Part model, mm, in its own coordinate system. Face numbers are marked on the shaded views. A direction names the side the tool comes from. Give positions to 0.01 mm unless a question says otherwise; leave off trailing zeros. Order: outer loops, then holes, each group sorted by start corner. A loop starts at its lowest first (then second) coordinate and runs counter-clockwise, first axis right, second up. Notation, with made-up numbers: (3, -11.5) - (28, -11.5) arc R21 cw to (28, 4.5) - close; hole circle Ø7 at (-21, -15). An arc over 180 degrees is marked (long way). One line per item, written item: value.
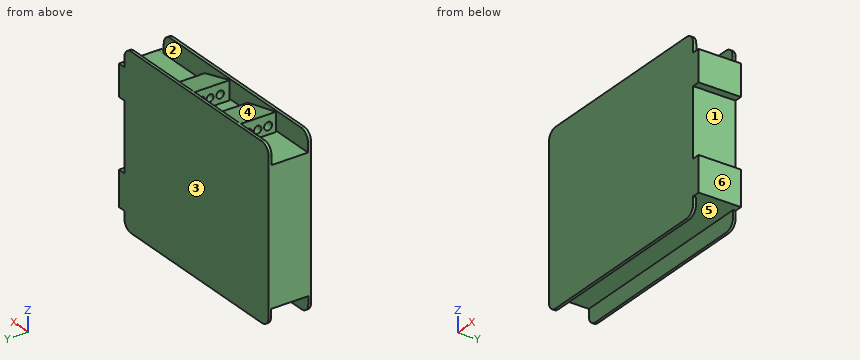
```python
from build123d import *

# Parameters (mm, degrees)
F1_DEPTH  = 22.5
F2_W      = 19.3578329636
F2_H      = 6.3240909576
F2_H_2    = 5.0115762651
F2_W_2    = 19.7066257242
F2_H_3    = 3.8353008032
F2_H_4    = 6.6283914447
F3_DEPTH  = 155.21203
F5_DEPTH  = 18.63889
F6_R      = 2.0341510362
F6_R_2    = 1.9663944792
F6_R_3    = 2.1232474026
F7_DEPTH  = 10
F8_R      = 2.0166596657
F8_R_2    = 1.8228540719
F8_R_3    = 1.9926186892
F9_DEPTH  = 10
F11_DEPTH = 5.64108
F13_DEPTH = 40.33136
F12_W     = 4
F12_H     = 18.4578578919
F12_H_2   = 17.5
F14_DEPTH = 25
F16_W     = 1.5692119678
F16_H     = 22.5
F17_DEPTH = 78.97005
F18_DEPTH = 25
F19_DEPTH = 25


with BuildPart() as f1:
    # F0 (on Front) → F1 (new body)
    with BuildSketch(Plane.XZ):
        with BuildLine():
            ThreePointArc((-43.9944155514, -30.0488834083), (-42.5299494574, -33.5844173142), (-38.9944155514, -35.0488834083))
            Line((-38.9944155514, -35.0488834083), (59.0055844486, -35.0488834083))
            ThreePointArc((59.0055844486, -35.0488834083), (62.5411183545, -33.5844173142), (64.0055844486, -30.0488834083))
            Line((64.0055844486, -30.0488834083), (64.0055844486, 49.9511165917))
            ThreePointArc((64.0055844486, 49.9511165917), (62.5411183545, 53.4866504976), (59.0055844486, 54.9511165917))
            Line((59.0055844486, 54.9511165917), (-38.9944155514, 54.9511165917))
            ThreePointArc((-38.9944155514, 54.9511165917), (-42.5299494574, 53.4866504976), (-43.9944155514, 49.9511165917))
            Line((-43.9944155514, 49.9511165917), (-43.9944155514, -30.0488834083))
        make_face()
    extrude(amount=F1_DEPTH)

    # F2 (on face) → F3 (cut)
    with BuildSketch(Plane(origin=(-43.9944155514, 0, 0), x_dir=(0, -1, 0), z_dir=(-1, 0, 0))):
        with Locations((11.1899548792, 53.1131620705)):
            Rectangle(F2_W, F2_H)
        with Locations((11.1899548792, 47.4453284591)):
            Rectangle(F2_W, F2_H_2)
        with Locations((11.1899542389, -28.1312330067)):
            Rectangle(F2_W_2, F2_H_3)
        with Locations((11.1899542389, -33.3630791306)):
            Rectangle(F2_W_2, F2_H_4)
    extrude(amount=-F3_DEPTH, mode=Mode.SUBTRACT)

    # F4 (on face) → F5 (join)
    with BuildSketch(Plane.XZ.offset(1.5110383974)):
        Polygon((0, 49.9453284591), (-21.0268571973, 54.9511165917), (-21.0268571973, 44.9395403266), (0, 44.9395403266), align=None)
        Polygon((32.1980565786, 49.9453284591), (13.5992644355, 54.9511165917), (13.5992644355, 44.9395403266), (32.1980565786, 44.9395403266), align=None)
    extrude(amount=F5_DEPTH)

    # F6 (on face) → F7 (cut)
    with BuildSketch(Plane(origin=(-21.0268571973, 0, 0), x_dir=(0, -1, 0), z_dir=(-1, 0, 0))):
        with Locations((5.4616648704, 49.1789467633)):
            Circle(F6_R)
        with Locations((10.4407919571, 49.1789467633)):
            Circle(F6_R_2)
        with Locations((15.9926619381, 49.1789467633)):
            Circle(F6_R_3)
    extrude(amount=-F7_DEPTH, mode=Mode.SUBTRACT)

    # F8 (on face) → F9 (cut)
    with BuildSketch(Plane(origin=(13.5992644355, 0, 0), x_dir=(0, -1, 0), z_dir=(-1, 0, 0))):
        with Locations((5.1434063353, 49.4216457009)):
            Circle(F8_R)
        with Locations((9.7698038444, 49.4216457009)):
            Circle(F8_R_2)
        with Locations((15.0747206062, 49.4216457009)):
            Circle(F8_R_3)
    extrude(amount=-F9_DEPTH, mode=Mode.SUBTRACT)

    # F10 (on face) → F11 (join)
    with BuildSketch(Plane.YZ.offset(64.0055844486)):
        Polygon((-20.868871361, 44.9503771961), (-22.5, 44.9503771961), (-22.5, 28.3550862223), (0, 28.3550862223), (0, 44.9503771961), (-1.5110383974, 44.9503771961), (-1.5110383974, 44.9395403266), (-20.868871361, 44.9395403266), align=None)
        Polygon((0, -8.5606295615), (-22.5, -8.5606295615), (-22.5, -26.2135826051), (-21.043267101, -26.2135826051), (-1.3366413768, -26.2135826051), (0, -26.2135826051), align=None)
    extrude(amount=F11_DEPTH)

    # F13 (add): a face of the model
    f13_faces = [f1.faces().sort_by_distance(p)[0] for p in [
        (66.8261244486, -11.25, 28.3550862223),
    ]]
    extrude(f13_faces, amount=F13_DEPTH)

    # F12 (on face) → F14 (cut)
    with BuildSketch(Plane.XZ.offset(22.5)):
        with Locations((66.0055844486, 19.1261572763)):
            Rectangle(F12_W, F12_H)
        with Locations((66.0055844486, 1.1472283304)):
            Rectangle(F12_W, F12_H_2)
    extrude(amount=-F14_DEPTH, mode=Mode.SUBTRACT)

    # F16 (on face) → F17 (cut)
    with BuildSketch(Plane(origin=(0, 0, -26.2135826051), x_dir=(1, 0, 0), z_dir=(0, 0, -1))):
        with Locations((68.8620584647, 11.25)):
            Rectangle(F16_W, F16_H)
    extrude(amount=-F17_DEPTH, mode=Mode.SUBTRACT)

    # F15 (on face) → F18 (cut)
    with BuildSketch(Plane(origin=(68.0055844486, 0, 0), x_dir=(0, -1, 0), z_dir=(-1, 0, 0))):
        Polygon((0, -7.6027716696), (22.0939440089, -7.6027716696), (21.3063190472, 28.3550862223), (0, 28.3550862223), align=None)
    extrude(amount=-F18_DEPTH, mode=Mode.SUBTRACT)

    # F19 (cut): a face of the model
    f19_faces = [f1.faces().sort_by_distance(p)[0] for p in [
        (68.0415184647, -21.7001315281, 10.3761572763),
    ]]
    extrude(f19_faces, amount=-F19_DEPTH, mode=Mode.SUBTRACT)


solid = f1.part
```
1) Pin check, flat tips, straight feed: pin 1 (4 mm diameter, centred on x = -25.5, z = 33.5, fed in from +Y); pin 2 (6.5 mm diameter, centred on y = -15.07, z = 49.42, fed in from -X); pin 3 (0.8 mm diameter, centred on x = 65.5, y = -0.5, fed in from +Z); pin 4 (6 mm diameter, centred on x = 2, y = -12, fed in from +Z). Stop position of each tip, or through.
Outcome:
pin 1: stops at y = 0
pin 2: stops at x = -21.03
pin 3: stops at z = 44.95
pin 4: stops at z = 50.18
2) Cut at B-B, the plane z = 23.5. Give the cut face in (x, y).
Outcome:
outline: (-43.99, -22.5) - (64.01, -22.5) - (64.01, 0) - (-43.99, 0) - close
3) Which spindle directions (+Z, -Z, +X, -X, +Y, -Y) get a long thin tool onto all of the face, cutting with end or side? Do the marked faces 1, 2 and 3. Say none if no direction does.
Outcome:
face 1: +X, +Y, -Y
face 2: +Z, +X, -X
face 3: +Z, -Z, +X, -X, +Y
4) Mould opens along X. For the marked faces 4, 5 and 6 say: released by +X, released by -X, zero draft, split by the parting line, or undercut.
Outcome:
face 4: undercut
face 5: zero draft
face 6: released by +X
5) Cut at A-A, the plane x = 5. Give the cut face in (y, z).
Outcome:
outline: (-22.5, -35.05) - (-21.04, -35.05) - (-21.04, -26.21) - (-1.34, -26.21) - (-1.34, -35.05) - (0, -35.05) - (0, 54.95) - (-1.51, 54.95) - (-1.51, 44.94) - (-20.87, 44.94) - (-20.87, 54.95) - (-22.5, 54.95) - close
6) Drill centre lines: line 1 along Y through (x, z) = (51, 50.5); line 2 along X through (y, z) = (-16, 7); line 3 along Z through (x, y) = (40, -18). Where is each one in solid material? Low to high. Write a range as from..to.
Outcome:
line 1: y = -22.5..-20.87, -1.51..0
line 2: x = -43.99..64.01
line 3: z = -26.21..44.94
